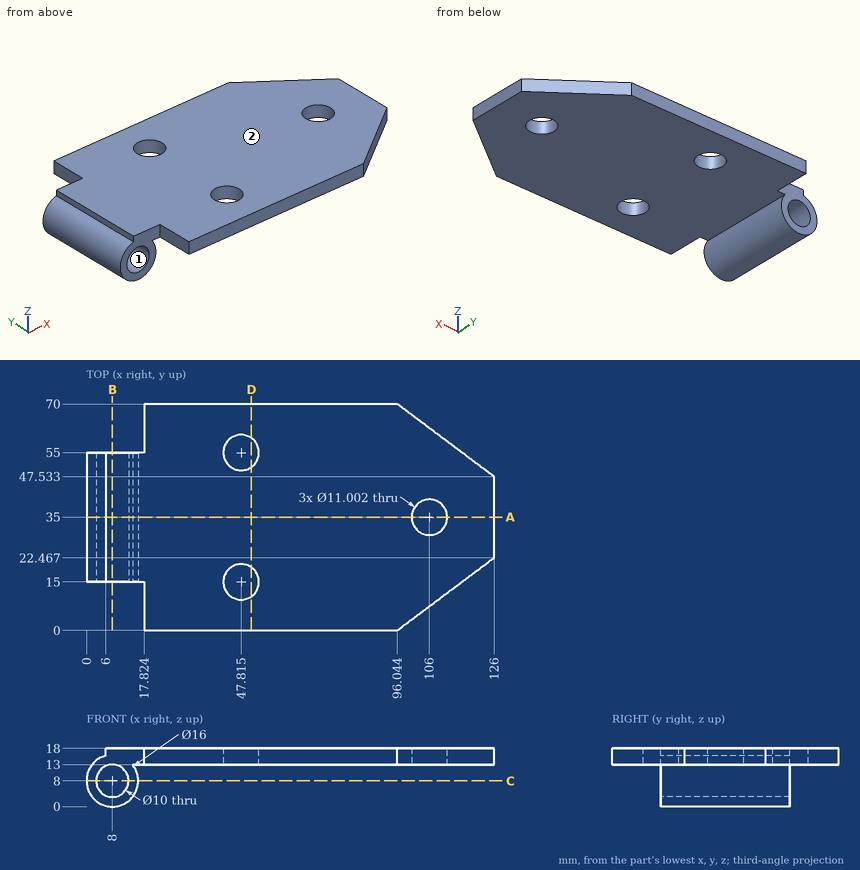
Geometry check sheet. Reference: drawing and pictorial views, mm from the part's lowest x, y, z. Give positions to 0.01 mm unless a question says otherwise; leave off trailing zeros. Write each loop counter-clockwise with the first axis right and the second up, starting at its lowest first coordinate (ties: lowest second). Pieces come first, ordered by that corner, then holes. Notation, with made-up numbers: M 57,-15 L 91,-15 A3 cw 91,-10 Z; hole C 28.25,-34 d6. An arc over 180 degrees is marked long. Put each result on its own line as item: value. Start each with the question number.
1. Section check B-B (x = 8). Record the cut outline in (y, z).
2. Section check D-D (x = 51). Record the cut outline in (y, z) (1 decimal), and give its area (3 significant figures).
3. Go/stop test with flat-tipped pins: pin 1 Ø9 at (x, z) = (12, 9.5) entering from +Y; pin 2 Ø1 at (y, z) = (41, 3) entering from +X (1 decimal); pin 3 Ø12.5 at (x, y) = (47.81, 55) entering from +Z; pin 4 Ø8 at (y, z) = (20.5, 3.5) entering from +X. Record where each tip stops, or that it passes through.
4. Section check C-C (z = 8). Record the cut outline in (x, y).
5. Draft check along X on the marked faces 1 and 2. Enter one of: +X half, -X half, draft (parallel to the pull), parting line (faces both ways), or undercut.
6. Scan lines: line 1 along X through (y, z) = (41, 8); line 2 along Z through (x, y) = (34.5, 25); line 3 along X through (y, z) = (17, 3.5) (1 decimal). Record each from-to range of solid material in increasing order. Write a range as [from, to].
7. Section check A-A (y = 35). Record the cut outline in (x, z) (1 decimal).
Answer list:
1. outline: M 15,0 L 55,0 L 55,3 L 15,3 Z; M 15,13 L 55,13 L 55,18 L 15,18 Z
2. outline: M 0,13 L 10.5,13 L 10.5,18 L 0,18 Z; M 19.5,13 L 50.5,13 L 50.5,18 L 19.5,18 Z; M 59.5,13 L 70,13 L 70,18 L 59.5,18 Z
2. area: 260 mm2
3. pin 1: y = 55
3. pin 2: x = 14.6
3. pin 3: z = 18
3. pin 4: x = 15.98
4. outline: M 0,15 L 3,15 L 3,55 L 0,55 Z; M 13,15 L 16,15 L 16,55 L 13,55 Z
5. face 1: undercut
5. face 2: draft
6. line 1: [0, 3], [13, 16]
6. line 2: [13, 18]
6. line 3: [1.4, 5.8], [10.2, 14.6]
7. outline: M 6,15.7 A8 ccw long 14.2,13 L 100.5,13 L 100.5,18 L 6,18 Z; M 111.5,13 L 126,13 L 126,18 L 111.5,18 Z; hole C 8,8 d10
